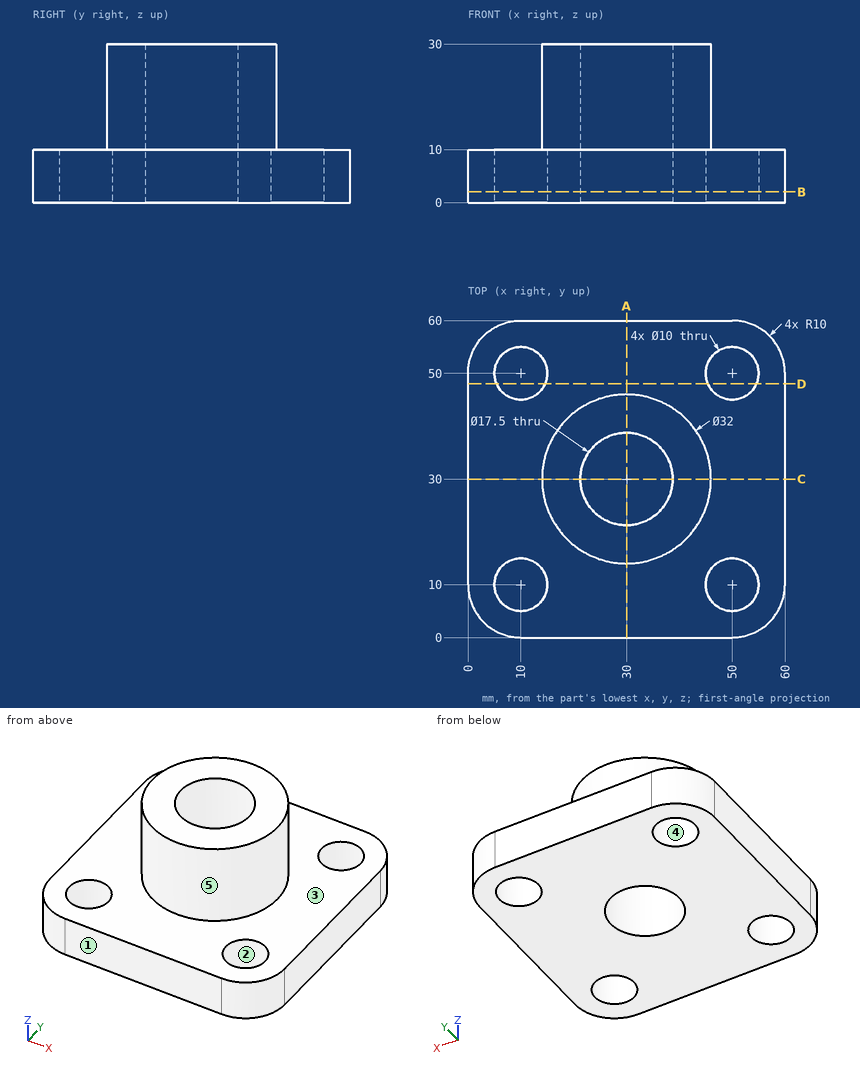
Here's the drawing with two shaded views (mm, measured from the low corner). I have some questions. A direction names the side the tool comes from. Coordinates: 2 decimals unless noted, no trailing zeros. Loops run counter-clockwise (first coordinate to the right, second up) from the corner with the lowest first, then second, coordinate; pieces in that order, holes last. Notation, with made-up numbers: M -30,57 L 5,57 A19 ccw 5,78 Z; hole C 15.25,48.25 d6. An arc over 180 degrees is marked long. Put each result on its own line as item: value. Start each with the question number.
(1) Imagine slicing it at B-B on z = 2. List the corners of the cut face in (x, y) for me.
(2) Imagine slicing it at D-D on y = 48. List the corners of the cut face in (x, z) for me.
(3) I need wall thicknesses on probe 1 along Y at (x, z) = (10, 2.25); probe 2 along Y at (x, z) = (30, 14.75). Which ranges of each line are inside material? Lowest first, please.
(4) Which directions (+Z, -Z, +X, -X, +Y, -Y) give clear straight access to the entire face, cutting with the end or side of a thin tool? Please do the marked faces 4 and 5.
(5) Imagine slicing it at A-A on x = 30. List the corners of the cut face in (y, z) for me, and give its area (3 significant figures).
(6) We'd pull the mould along Y, two halves only. Please class the marked faces 1, 2 and 3: +Y half, -Y half, draft (parallel to the pull), parting line (faces both ways), or undercut.
(7) Will these pins go through, and if not, where does the flat tip stop? pin 1 Ø12 at (y, z) = (32, 24) entering from +X; pin 2 Ø5 at (x, z) = (28.5, 6) entering from -Y; pin 3 Ø8 at (x, z) = (22.5, 24.5) entering from -Y; pin 4 Ø13 at (x, y) = (50, 50) entering from +Z.
Worked answers:
1. outline: M 0,10 A10 ccw 10,0 L 50,0 A10 ccw 60,10 L 60,50 A10 ccw 50,60 L 10,60 A10 ccw 0,50 Z; hole C 10,10 d10; hole C 10,50 d10; hole C 30,30 d17.5; hole C 50,10 d10; hole C 50,50 d10
2. outline: M 0,0 L 5.42,0 L 5.42,10 L 0,10 Z; M 14.58,0 L 45.42,0 L 45.42,10 L 14.58,10 Z; M 54.58,0 L 60,0 L 60,10 L 54.58,10 Z
3. probe 1: y = 0 to 5, 15 to 45, 55 to 60
3. probe 2: y = 14 to 21.25, 38.75 to 46
4. face 4: +Z, -Z
4. face 5: +Z
5. outline: M 0,0 L 21.25,0 L 21.25,30 L 14,30 L 14,10 L 0,10 Z; M 38.75,0 L 60,0 L 60,10 L 46,10 L 46,30 L 38.75,30 Z
5. area: 715 mm2
6. face 1: -Y half
6. face 2: undercut
6. face 3: draft
7. pin 1: stops at x = 46
7. pin 2: stops at y = 0
7. pin 3: stops at y = 14.39
7. pin 4: stops at z = 10
